Geometry check sheet. Reference: drawing and pictorial views, mm from the part's lowest x, y, z. A direction names the side the tool comes from. Round coordinates to 2 decimals unless told otherwise and drop trailing zeros. Order: outer loops, then holes, each group sorted by start corner. A loop starts at its lowest first (then second) coordinate and runs counter-clockwise, first axis right, second up.
(1) Depth check by flat-ended pin: pin 1 (1.5 mm diameter, centred on y = 25, z = 24, fed in from -X); pin 2 (6.5 mm diameter, centred on x = 7, z = 9, fed in from +Y); pin 3 (2 mm diameter, centred on y = 41.5, z = 22, fed in from +X); pin 4 (1.7 mm diameter, centred on x = 13, y = 40, fed in from -Z). Enter the tip coordinate at first touch or a pass-through.
(2) Tool access check on the marked faces 1 and 2. Record the directions out of +Z, -Z, +X, -X, +Y, -Y that give a thin tool (end or side, any length) a straight path to the whole face; none if there is none.
(3) Mould release check, pull along Y, two halves, no side actions. Record for the marked faces 3, 4, 5 and 6: released by +Y, released by -Y, zero draft, split by the parting line, or undercut.
(4) Sectioned sample at D-D, the plane z = 11.5. Enter the section's corners in (x, y), and give its area (3 significant figures).
(5) Thickness scan on probe 1 along X at (y, z) = (2, 7.5); probe 2 along Z at (x, y) = (18, 33); probe 3 along Y at (x, z) = (5.5, 22). Record the ranges inside material, lowest first.
(6) Sectioned sample at B-B, the plane x = 4. Enter the section's corners in (y, z).
(7) Sectioned sample at C-C, the plane y = 39. Enter the section's corners in (x, z).
(8) Sectioned sample at A-A, the plane x = 12.5. Enter the section's corners in (y, z), and give its area (4 significant figures).
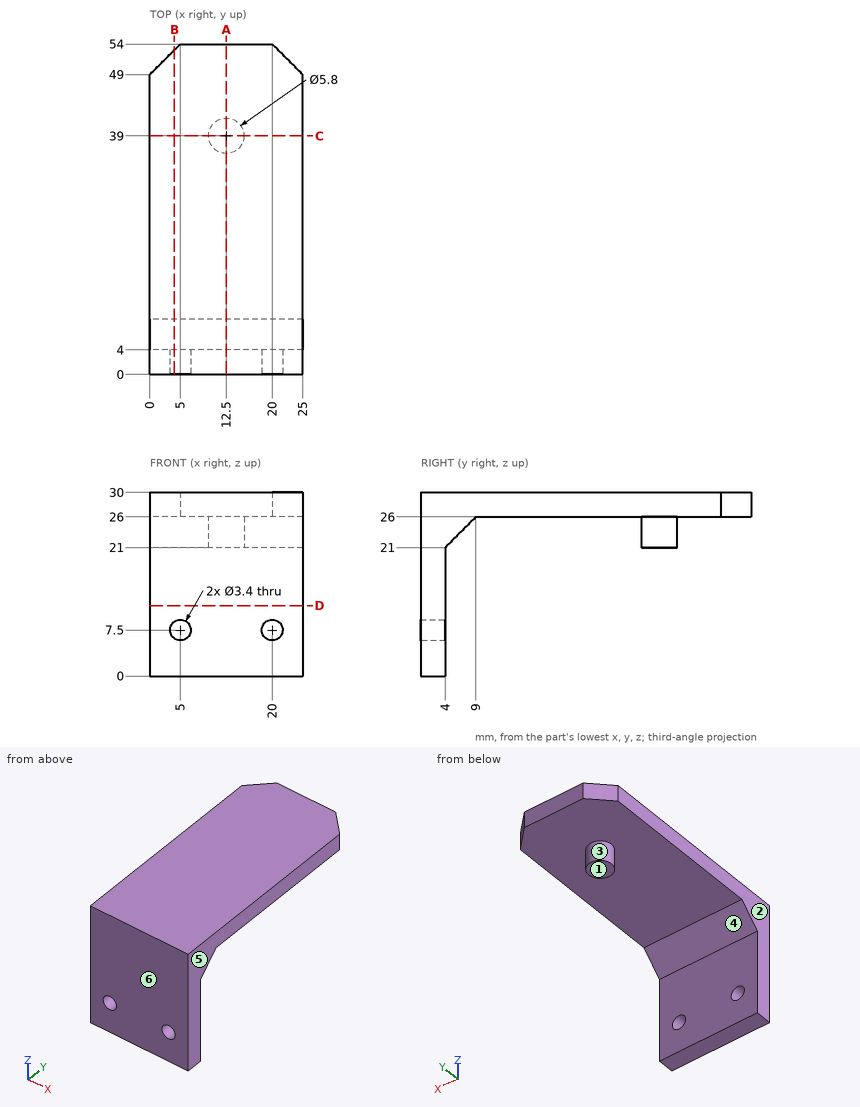
Derived:
1. pin 1: passes through
1. pin 2: stops at y = 4
1. pin 3: stops at x = 14.98
1. pin 4: stops at z = 21
2. face 1: -Z, +X, -X, +Y
2. face 2: +Z, -Z, -X, +Y, -Y
3. face 3: undercut
3. face 4: undercut
3. face 5: zero draft
3. face 6: released by -Y
4. outline: (0, 0) - (25, 0) - (25, 4) - (0, 4) - close
4. area: 100 mm2
5. probe 1: x = 0 to 3.3, 6.7 to 18.3, 21.7 to 25
5. probe 2: z = 26 to 30
5. probe 3: y = 0 to 5
6. outline: (0, 0) - (4, 0) - (4, 6.13) - (0, 6.13) - close; (0, 8.87) - (4, 8.87) - (4, 21) - (9, 26) - (53, 26) - (53, 30) - (0, 30) - close
7. outline: (0, 26) - (9.6, 26) - (9.6, 21) - (15.4, 21) - (15.4, 26) - (25, 26) - (25, 30) - (0, 30) - close
8. outline: (0, 0) - (4, 0) - (4, 21) - (9, 26) - (36.1, 26) - (36.1, 21) - (41.9, 21) - (41.9, 26) - (54, 26) - (54, 30) - (0, 30) - close
8. area: 361.5 mm2
